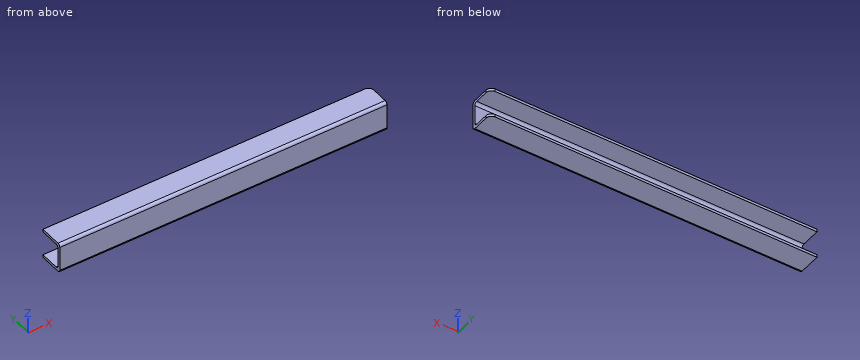
Autodesk Inventor part; units mm, degrees
ref_plane "YZ Plane" through (0, 0, 0) normal (1, 0, 0) x (0, 1, 0)
ref_plane "XZ Plane" through (0, 0, 0) normal (0, 1, 0) x (-1, 0, 0)
ref_plane "XY Plane" through (0, 0, 0) normal (0, 0, 1) x (1, 0, 0)
sketch "Sketch1" plane through (0, 0, 0) normal (0, 1, 0) x (-1, 0, 0)
  point P0 (0, 0)
sketch "Sketch2" plane through (0, 0, 0) normal (0, 1, 0) x (-1, 0, 0)
  line L0 (381, 15.875) -> (-381, 15.875)
  line L1 (-381, 15.875) -> (-381, -15.875)
  line L2 (-381, -15.875) -> (381, -15.875)
  line L3 (381, -15.875) -> (381, 15.875)
  point P0 (0, 0)
  dimension "d2" = 762
  dimension "d3" = 31.75
extrude "Extrusion1" add sketch "Sketch2" along normal blind 3.175
sketch "Sketch3" plane through (381, 0, -15.875) normal (0, 0, -1) x (-1, 0, 0)
  point P0 (381, 0)
sketch "Sketch4" plane through (0, 0, 0) normal (0, -1, 0) x (1, 0, 0)
  point P0 (0, 0)
sketch "Sketch5" plane through (0, 0, 0) normal (0, -1, 0) x (1, 0, 0)
  line L0 (381, -15.875) -> (-381, -15.875)
  line L1 (-381, -15.875) -> (-381, -19.05)
  line L2 (-381, -19.05) -> (381, -19.05)
  line L3 (381, -19.05) -> (381, -15.875)
  point P0 (0, 0)
  dimension "d6" = 762
  dimension "d7" = 3.175
extrude "Extrusion2" add sketch "Sketch5" against normal blind 3.175
sketch "Sketch6" plane through (-381, 0, 15.875) normal (0, 0, 1) x (1, 0, 0)
  line L0 (0, 0) -> (762, 0)
  line L1 (762, 0) -> (762, 28.575)
  line L2 (762, 28.575) -> (0, 28.575)
  line L3 (0, 28.575) -> (0, 0)
  point P0 (381, 0)
  dimension "d10" = 762
  dimension "d11" = 28.575
sketch "Sketch7" plane through (0, 3.175, 0) normal (0, 1, 0) x (1, 0, 0)
  line L0 (-381, -15.875) -> (381, -15.875)
  line L1 (381, -15.875) -> (381, -12.7)
  line L2 (381, -12.7) -> (-381, -12.7)
  line L3 (-381, -12.7) -> (-381, -15.875)
  point P0 (0, 0)
  dimension "d12" = 762
  dimension "d13" = 3.175
extrude "Extrusion3" cut sketch "Sketch7" against normal blind 3.175
extrude "Extrusion4" add sketch "Sketch6" against normal blind 3.175
sketch "Sketch8" plane through (0, 3.175, 0) normal (0, 1, 0) x (1, 0, 0)
  point P0 (0, 0)
sketch "Sketch9" plane through (381, 0, -19.05) normal (0, 0, -1) x (-1, 0, 0)
  line L0 (0, 0) -> (762, 0)
  line L1 (762, 0) -> (762, 28.575)
  line L2 (762, 28.575) -> (0, 28.575)
  line L3 (0, 28.575) -> (0, 0)
  point P0 (381, 0)
  dimension "d18" = 762
  dimension "d19" = 28.575
sketch "Sketch10" plane through (0, 3.175, 0) normal (0, 1, 0) x (1, 0, 0)
  line L0 (381, 19.05) -> (-381, 19.05)
  line L1 (-381, 19.05) -> (-381, 15.875)
  line L2 (-381, 15.875) -> (381, 15.875)
  line L3 (381, 15.875) -> (381, 19.05)
  point P0 (0, 0)
  dimension "d20" = 762
  dimension "d21" = 3.175
extrude "Extrusion5" cut sketch "Sketch10" against normal blind 3.175
extrude "Extrusion6" add sketch "Sketch9" against normal blind 3.175
fillet "Fillet1" radius 3.175 1 edges at (0, 3.175, 12.7)
fillet "Fillet2" radius 3.175 1 edges at (0, 3.175, -15.875)
fillet "Fillet3" radius 3.175 1 edges at (0, 0, 15.875)
fillet "Fillet4" radius 3.175 1 edges at (0, 0, -19.05)
fillet "Fillet5" radius 6.35 1 edges at (-381, 28.575, -17.4625)
fillet "Fillet6" radius 6.35 1 edges at (-381, 28.575, 14.2875)
fillet "Fillet7" radius 6.35 1 edges at (381, 28.575, 14.2875)
fillet "Fillet8" radius 6.35 1 edges at (381, 28.575, -17.4625)
sketch "Sketch11" plane through (0, 3.175, 0) normal (0, 1, 0) x (1, 0, 0)
  point P0 (0, 0)
sketch "Sketch12" plane through (0, 0, 0) normal (0, -1, 0) x (1, 0, 0)
  line L0 (374.65, 15.875) -> (-374.65, 15.875)
  line L1 (0, 15.875) -> (-381, 15.875)
  line L2 (-381, 15.875) -> (-381, -19.05)
  line L3 (-381, -19.05) -> (0, -19.05)
  line L4 (0, -19.05) -> (0, 15.875)
  point P0 (0, 0)
extrude "Extrusion7" cut sketch "Sketch12" against normal blind 28.575
properties part number "alignmentWheelsBar"
Verification items for the finished model (mm, model axes). Give positions to 0.01 mm unless a question says otherwise; leave off trailing zeros. Loops run counter-clockwise (first coordinate to the right, second up) from the corner with the lowest first, then second, coordinate; pieces in that order, holes last.
1. Thickness scan on line 1 (Z direction, x = 333, y = 20.5) (3 decimals); line 2 (Y direction, x = 94, z = 7) (3 decimals); line 3 (Z direction, x = 131.5, y = 4) (3 decimals). Record the ranges inside material, lowest first.
2. Section check C-C, the plane z = 4. Enter the section's corners in (x, y) (3 decimals), then the cut area to 3 significant figures.
3. Go/stop test with a flat-tipped pin: pin 1 Ø1 at (x, z) = (329.5, 9.5) entering from +Y. Record where the tip stops, or that it passes through.
4. Section check B-B, the plane x = 144.5. Enter the section's corners in (y, z) (3 decimals), then the cut area to 3 significant figures.
5. Section check A-A, the plane y = 11. Enter the section's corners in (x, z) (3 decimals), then the cut area to 3 significant figures.
Geometry says:
1. line 1: z = -19.05 to -15.875, 12.7 to 15.875
1. line 2: y = 0 to 3.175
1. line 3: z = -19.05 to -14.835, 11.66 to 15.875
2. outline: (0, 0) - (381, 0) - (381, 3.175) - (0, 3.175) - close
2. area: 1,210 mm2
3. pin 1: stops at y = 3.21
4. outline: (0, -15.875) arc R3.175 ccw to (3.175, -19.05) - (28.575, -19.05) - (28.575, -15.875) - (6.35, -15.875) arc R3.175 cw to (3.175, -12.7) - (3.175, 9.525) arc R3.175 cw to (6.35, 12.7) - (28.575, 12.7) - (28.575, 15.875) - (3.175, 15.875) arc R3.175 ccw to (0, 12.7) - close
4. area: 272 mm2
5. outline: (0, -19.05) - (381, -19.05) - (381, -15.875) - (0, -15.875) - close; (0, 12.7) - (381, 12.7) - (381, 15.875) - (0, 15.875) - close
5. area: 2,420 mm2
